Verification items for the finished model (mm, model axes). A direction names the side the tool comes from. Coordinates: 2 decimals unless noted, no trailing zeros. Loops run counter-clockwise (first coordinate to the right, second up) from the corner with the lowest first, then second, coordinate; pieces in that order, holes last.
Q1. Sectioned sample at B-B (x = 0). Enter the section's corners in (y, z).
Q2. Go/stop test with flat-tipped pins: P1, Ø6, axis at x = -7.5, z = -33.5, coming from the -Y side; P2, Ø6, axis at x = 1.5, y = 7.5, coming from the +Z side; P3, Ø2, axis at x = 2, y = 5.5, coming from the +Z side; P4, Ø3, axis at x = 9.5, z = -27.5, coming from the +Y side. Record where each tip stops, or that it passes through.
Q3. Access from +Z, -Z, +X, -X, +Y, -Y to the whole of each face (thin tool, end or side, straight path). Record for faces 4 (the face through (9.35, 6.64, -4.762)), 5 (the face through (3, -8, -1.588)), 6 (the face through (0, 0, -76.2)).
Q4. Mould release check, pull along Z, two halves, no side actions. Record for faces 1 (the face through (9.35, -6.64, -7.938)), 2 (the face through (0, 0, -25.4)), 3 (the face through (-1.72, -7.75, -7.07)): +Z half, -Z half, draft (parallel to the pull), parting line (faces both ways), or undercut.
Q5. Material ranges on probe 1 along Z at (x, y) = (2.5, -11.25); probe 2 along Y at (x, z) = (0, -3.75); probe 3 along Y at (x, z) = (0, -17), recorded low to high.
Q6. Sectioned sample at A-A (y = 5.5). Enter the section's corners in (x, z).
Q7. Sectioned sample at D-D (y = -9.5). Enter the section's corners in (x, z).
Q8. Sectioned sample at C-C (z = -67). Enter the section's corners in (x, y), then the cut area to 3 significant figures.
```python
from build123d import *

# Parameters (mm, degrees)
F2_R     = 7.9375
F2_R_2   = 4.7625
F3_DEPTH = 12.7
F4_R     = 10.31875
F4_R_2   = 7.9375
F5_DEPTH = 1.5875


with BuildPart() as f1:
    # F0 (on Right) → F1 (revolve)
    with BuildSketch(Plane.YZ):
        Polygon((12.7, -4.7625), (12.7, 0), (4.7625, 0), (4.7625, -25.4), (0, -25.4), (0, -76.2), (12.7, -76.2), (12.7, -7.9375), (11.265334, -7.9375), (11.265334, -4.7625), align=None)
    revolve(axis=Axis((0, 0, -33.687185), (0, 0, 1)))

    # F2 (on face) → F3 (cut)
    with BuildSketch(Plane.XY):
        Circle(F2_R)
        Circle(F2_R_2, mode=Mode.SUBTRACT)
    extrude(amount=-F3_DEPTH, mode=Mode.SUBTRACT)

    # F4 (on face) → F5 (cut)
    with BuildSketch(Plane.XY):
        Circle(F4_R)
        Circle(F4_R_2, mode=Mode.SUBTRACT)
    extrude(amount=-F5_DEPTH, mode=Mode.SUBTRACT)


solid = f1.part
```
Geometry check:
1. outline: (-12.7, -76.2) - (12.7, -76.2) - (12.7, -7.94) - (11.27, -7.94) - (11.27, -4.76) - (12.7, -4.76) - (12.7, 0) - (10.32, 0) - (10.32, -1.59) - (7.94, -1.59) - (7.94, -12.7) - (4.76, -12.7) - (4.76, -25.4) - (-4.76, -25.4) - (-4.76, -12.7) - (-7.94, -12.7) - (-7.94, -1.59) - (-10.32, -1.59) - (-10.32, 0) - (-12.7, 0) - (-12.7, -4.76) - (-11.27, -4.76) - (-11.27, -7.94) - (-12.7, -7.94) - close
2. P1: stops at y = -11.88
2. P2: stops at z = 0
2. P3: stops at z = -12.7
2. P4: stops at y = 9.86
3. face 4: none
3. face 5: +Z
3. face 6: -Z, +X, -X, +Y, -Y
4. face 1: undercut
4. face 2: +Z half
4. face 3: draft
5. probe 1: z = -76.2 to -7.94, -4.76 to 0
5. probe 2: y = -12.7 to -7.94, 7.94 to 12.7
5. probe 3: y = -12.7 to -4.76, 4.76 to 12.7
6. outline: (-11.45, -76.2) - (11.45, -76.2) - (11.45, -7.94) - (9.83, -7.94) - (9.83, -4.76) - (11.45, -4.76) - (11.45, 0) - (8.73, 0) - (8.73, -1.59) - (5.72, -1.59) - (5.72, -12.7) - (-5.72, -12.7) - (-5.72, -1.59) - (-8.73, -1.59) - (-8.73, 0) - (-11.45, 0) - (-11.45, -4.76) - (-9.83, -4.76) - (-9.83, -7.94) - (-11.45, -7.94) - close
7. outline: (-8.43, -76.2) - (8.43, -76.2) - (8.43, -7.94) - (6.05, -7.94) - (6.05, -4.76) - (8.43, -4.76) - (8.43, 0) - (4.03, 0) - (4.03, -1.59) - (-4.03, -1.59) - (-4.03, 0) - (-8.43, 0) - (-8.43, -4.76) - (-6.05, -4.76) - (-6.05, -7.94) - (-8.43, -7.94) - close
8. outline: circle Ø25.4 at (0, 0)
8. area: 507 mm2
